CAD build for the part. Positions are in the model's coordinates, mm. A direction names the side the tool comes from. Coordinates: 2 decimals unless noted, no trailing zeros. Order: outer loops, then holes, each group sorted by start corner. A loop starts at its lowest first (then second) coordinate and runs counter-clockwise, first axis right, second up. Notation, with made-up numbers: (45, 1.5) - (78, 1.5) arc R13 ccw to (78, 19.5) - close; hole circle Ø8 at (41, 81.5). An arc over 180 degrees is marked (long way). Return JSON: item names as keys, results as strings.
from build123d import *

# Parameters (mm, degrees)
SKETCH_1_W          = 95
SKETCH_1_H          = 120
EXTRUDE_1_DEPTH     = 3
SKETCH_2_W          = 3
SKETCH_2_H          = 37.7
EXTRUDE_2_DEPTH     = 70
SKETCH_3_W          = 39.9
SKETCH_3_H          = 19.7
SKETCH_3_R          = 2.1
CUT_EXTRUDE_1_DEPTH = 61
SKETCH_4_R          = 1.5
CUT_EXTRUDE_2_DEPTH = 10
SKETCH_5_W          = 56.6
SKETCH_5_H          = 19.7
EXTRUDE_3_DEPTH     = 3
SKETCH_6_W          = 56.6
SKETCH_6_H          = 39.9
EXTRUDE_4_DEPTH     = 3
EXTRUDE_5_DEPTH     = 3
SKETCH_9_W          = 12
SKETCH_9_H          = 12
EXTRUDE_6_DEPTH     = 3
SKETCH_10_W         = 39.9
SKETCH_10_H         = 9
CUT_EXTRUDE_4_DEPTH = 74
SKETCH_13_W         = 56.6
SKETCH_13_H         = 10
CUT_EXTRUDE_5_DEPTH = 14


with BuildPart() as part:
    # 草图1 → 凸台-拉伸1 (new body)
    with BuildSketch(Plane.XY):
        with Locations((-42.5, 0.779220779)):
            Rectangle(SKETCH_1_W, SKETCH_1_H)
    extrude(amount=EXTRUDE_1_DEPTH)

    # 草图2 → 凸台-拉伸2 (add)
    with BuildSketch(Plane(origin=(0, 0, 0), x_dir=(-1, 0, 0), z_dir=(0, 0, -1))):
        with Locations((15.7, 0.779220779)):
            Rectangle(SKETCH_2_W, SKETCH_2_H)
        with Locations((69.3, 0.779220779)):
            Rectangle(SKETCH_2_W, SKETCH_2_H)
    extrude(amount=EXTRUDE_2_DEPTH)

    # 草图3 → 切除-拉伸1 (cut)
    with BuildSketch(Plane(origin=(-14.2, 0, 0), x_dir=(0, 0, -1), z_dir=(1, 0, 0))):
        with Locations((41.05, 0.779220779)):
            Rectangle(SKETCH_3_W, SKETCH_3_H)
        with Locations((16.34, -4.145779221)):
            Circle(SKETCH_3_R)
        with Locations((65.76, 5.704220779)):
            Circle(SKETCH_3_R)
        with Locations((65.76, -4.145779221)):
            Circle(SKETCH_3_R)
        with Locations((16.34, 5.704220779)):
            Circle(SKETCH_3_R)
    extrude(amount=-CUT_EXTRUDE_1_DEPTH, mode=Mode.SUBTRACT)

    # 草图4 → 切除-拉伸2 (cut)
    with BuildSketch(Plane.XY.offset(3)):
        with Locations((-75, 57.779220779)):
            Circle(SKETCH_4_R)
        with Locations(Location((-10, 57.779220779, 0), (0, 0, 180))):
            Circle(SKETCH_4_R)
        with Locations((-10, -56.220779221)):
            Circle(SKETCH_4_R)
        with Locations(Location((-75, -56.220779221, 0), (0, 0, 180))):
            Circle(SKETCH_4_R)
    extrude(amount=-CUT_EXTRUDE_2_DEPTH, mode=Mode.SUBTRACT)

    # 草图5 → 凸台-拉伸3 (add)
    with BuildSketch(Plane(origin=(0, 0, -70), x_dir=(-1, 0, 0), z_dir=(0, 0, -1))):
        with Locations((42.5, 0.779220779)):
            Rectangle(SKETCH_5_W, SKETCH_5_H)
    extrude(amount=EXTRUDE_3_DEPTH)

    # 草图6 → 凸台-拉伸4 (add)
    with BuildSketch(Plane(origin=(0, 19.629220779, 0), x_dir=(1, 0, 0), z_dir=(0, 1, 0))):
        with Locations((-42.5, 41.05)):
            Rectangle(SKETCH_6_W, SKETCH_6_H)
    extrude(amount=EXTRUDE_4_DEPTH)

    # 草图8 → 凸台-拉伸5 (add)
    with BuildSketch(Plane(origin=(-14.2, 0, 0), x_dir=(0, 0, -1), z_dir=(1, 0, 0))):
        Polygon((61, 22.629220779), (61, 19.629220779), (70, 19.629220779), (70, 10.629220779), (73, 10.629220779), (73, 22.629220779), align=None)
        Polygon((73, -9.070779221), (70, -9.070779221), (70, -18.070779221), (61, -18.070779221), (61, -21.070779221), (73, -21.070779221), align=None)
    extrude(amount=-EXTRUDE_5_DEPTH)

    # 草图9 → 凸台-拉伸6 (add)
    with BuildSketch(Plane.ZY.offset(70.8)):
        with Locations((-67, 16.629220779)):
            Rectangle(SKETCH_9_W, SKETCH_9_H)
        with Locations((-67, -15.070779221)):
            Rectangle(SKETCH_9_W, SKETCH_9_H)
    extrude(amount=-EXTRUDE_6_DEPTH)

    # 草图10 → 切除-拉伸4 (cut)
    with BuildSketch(Plane(origin=(-14.2, 0, 0), x_dir=(0, 0, -1), z_dir=(1, 0, 0))):
        Polygon((73, 10.629220779), (73, 22.629220779), (61, 22.629220779), align=None)
        Polygon((73, -9.070779221), (73, -21.070779221), (61, -21.070779221), align=None)
        with Locations((41.05, -13.570779221)):
            Rectangle(SKETCH_10_W, SKETCH_10_H)
    extrude(amount=-CUT_EXTRUDE_4_DEPTH, mode=Mode.SUBTRACT)

    # 草图13 → 切除-拉伸5 (cut)
    with BuildSketch(Plane(origin=(0, 0, 0), x_dir=(-1, 0, 0), z_dir=(0, 0, -1))):
        with Locations((42.5, 39.629220779)):
            Rectangle(SKETCH_13_W, SKETCH_13_H)
        with Locations((42.5, -38.070779221)):
            Rectangle(SKETCH_13_W, SKETCH_13_H)
    extrude(amount=-CUT_EXTRUDE_5_DEPTH, mode=Mode.SUBTRACT)


solid = part.part
Item 1: Band-saw the part on C-C, the plane x = -10. List the corners of the cut face in (y, z).
Findings below:
{"outline": "(-59.22, 0) - (-57.72, 0) - (-57.72, 3) - (-59.22, 3) - close; (-54.72, 0) - (56.28, 0) - (56.28, 3) - (-54.72, 3) - close; (59.28, 0) - (60.78, 0) - (60.78, 3) - (59.28, 3) - close"}
Item 2: Which spindle directions (+Z, -Z, +X, -X, +Y, -Y) get a long thin tool onto all of the face, cutting with end or side? Do faces 1 (the cylindrical face through (-69.279, 5.797, -63.662)), 2 (the flat face through (-16, -18.071, -10)), 3 (the flat face through (-70.8, -38, 1)). Say none if no direction does.
Findings below:
{"face 1": "+X, -X", "face 2": "+X, -X, -Y", "face 3": "+Z, -Z"}
Item 3: Wall check: L1, parallel to X at y = -1.5, z = -21; L2, parallel to Y at x = -75, z = 2; L3, parallel to Y at x = -15.5, z = -65.76. Give the ranges that are in metal, low to high. Write a range as [from, to].
Findings below:
{"L1": "x = [-70.8, -67.8], [-17.2, -14.2]", "L2": "y = [-59.22, -57.72], [-54.72, 56.28], [59.28, 60.78]", "L3": "y = [-16.31, -6.25], [-2.05, 3.6], [7.8, 17.87]"}
Item 4: Mould opens along X. For faces 4 (the flat face through (-67.8, 11, -37)), 5 (the cylindrical face through (-15.679, 5.797, -63.662)) say: released by +X, released by -X, zero draft, split by the parting line, or undercut.
Findings below:
{"face 4": "undercut", "face 5": "zero draft"}
Item 5: Band-saw the part on A-A, the plane y = 1. List the corners of the cut face in (x, z), then the cut area to 3 significant figures.
Findings below:
{"outline": "(-90, 0) - (-70.8, 0) - (-70.8, -21.1) - (-67.8, -21.1) - (-67.8, 0) - (-17.2, 0) - (-17.2, -21.1) - (-14.2, -21.1) - (-14.2, 0) - (5, 0) - (5, 3) - (-90, 3) - close; (-70.8, -73) - (-14.2, -73) - (-14.2, -61) - (-17.2, -61) - (-17.2, -70) - (-67.8, -70) - (-67.8, -61) - (-70.8, -61) - close", "area": "635 mm²"}
Item 6: Band-saw the part on D-D, the plane x = -32. List the corners of the cut face in (y, z).
Findings below:
{"outline": "(-59.22, 0) - (-43.07, 0) - (-43.07, 3) - (-59.22, 3) - close; (-33.07, 0) - (34.63, 0) - (34.63, 3) - (-33.07, 3) - close; (-9.07, -73) - (10.63, -73) - (10.63, -70) - (-9.07, -70) - close; (19.63, -61) - (22.63, -61) - (22.63, -21.1) - (19.63, -21.1) - close; (44.63, 0) - (60.78, 0) - (60.78, 3) - (44.63, 3) - close"}
Item 7: Drop flat-ended pins along their axis: P1, Ø6.5, axis at y = 5.7, z = -16.34, coming from the -X side; P2, Ø1.5, axis at x = -51.5, z = -32, coming from the -Y side; P3, Ø1.5, axis at x = -12.5, y = -35.5, coming from the -Z side. Give the stop position or say it passes through.
Findings below:
{"P1": "stops at x = -70.8", "P2": "stops at y = 19.63", "P3": "stops at z = 0"}
Item 8: Band-saw the part on B-B, the plane z = -16.34. List the corners of the cut face in (x, y).
Findings below:
{"outline": "(-70.8, -18.07) - (-67.8, -18.07) - (-67.8, -6.25) - (-70.8, -6.25) - close; (-70.8, -2.05) - (-67.8, -2.05) - (-67.8, 3.6) - (-70.8, 3.6) - close; (-70.8, 7.8) - (-67.8, 7.8) - (-67.8, 19.63) - (-70.8, 19.63) - close; (-17.2, -18.07) - (-14.2, -18.07) - (-14.2, -6.25) - (-17.2, -6.25) - close; (-17.2, -2.05) - (-14.2, -2.05) - (-14.2, 3.6) - (-17.2, 3.6) - close; (-17.2, 7.8) - (-14.2, 7.8) - (-14.2, 19.63) - (-17.2, 19.63) - close"}
